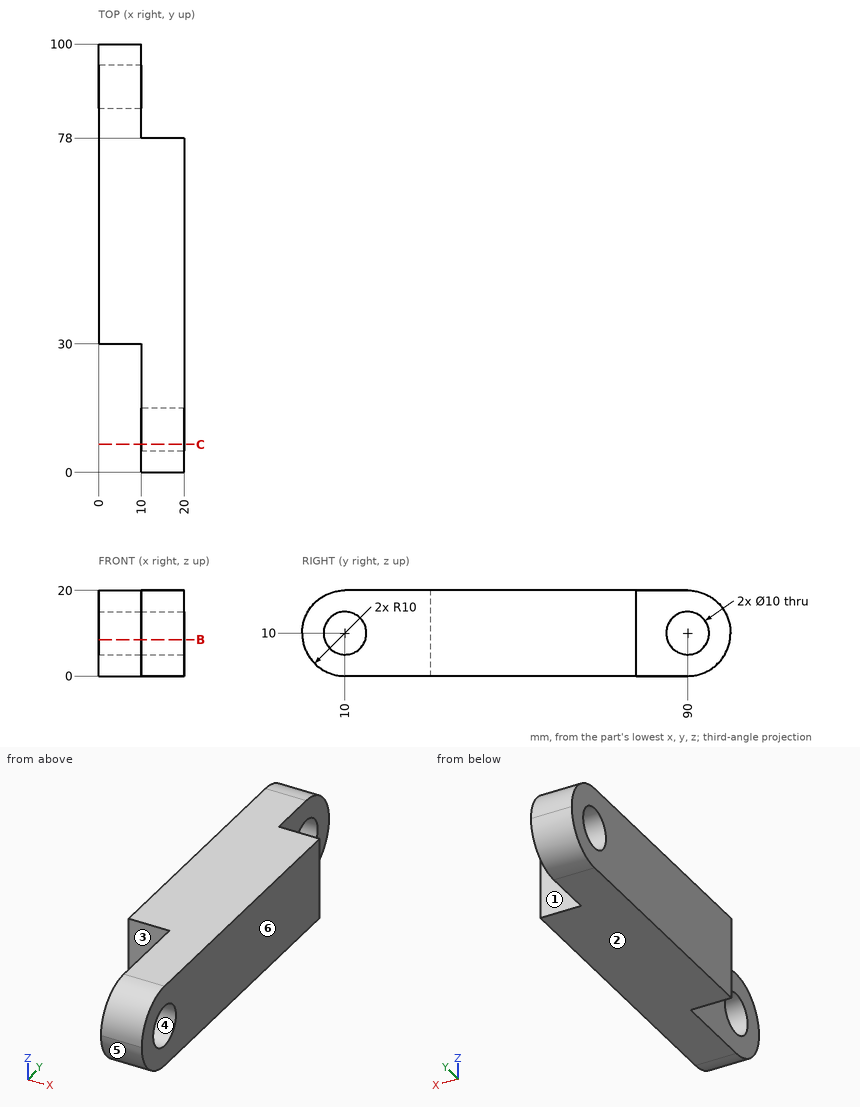
Can you work these out from the drawing? Everything is in mm from the part's minimum corner. A direction names the side the tool comes from. Round coordinates to 2 decimals unless told otherwise and drop trailing zeros. Order: outer loops, then holes, each group sorted by start corner. A loop starts at its lowest first (then second) coordinate and runs counter-clockwise, first axis right, second up. Notation, with made-up numbers: M -31,-37 L -7,-37 A25 cw -7,-21 Z; hole C -30,30.5 d3. An arc over 180 degrees is marked long. Answer as CSV lines item,"result".
Item 1: Imagine slicing it at C-C on y = 6.5. List the corners of the cut face in (x, z) for me.
From the geometry:
outline,"M 10,0.63 L 20,0.63 L 20,6.43 L 10,6.43 Z; M 10,13.57 L 20,13.57 L 20,19.37 L 10,19.37 Z"
Item 2: Please list where these lines run through material, in increasing order: L1, parallel to Z at x = 13.5, y = 10; L2, parallel to X at y = 82.5, z = 11.25; L3, parallel to Y at x = 4.75, z = 13. Write a range as [from, to].
From the geometry:
L1,"[0, 5], [15, 20]"
L2,"[0, 10]"
L3,"[30, 86], [94, 99.54]"
Item 3: For pin 1 (6 mm diameter, centred on y = 94, z = 13.5, fed in from +X); pin 2 (5 mm diameter, centred on x = 4, z = 15, fed in from -Y); pin 3 (8 mm diameter, centred on x = 6.5, z = 3.5, fed in from +Y), each with a flat end and sliding along its axis, tell me the tip position at first contact or that it passes through.
From the geometry:
pin 1,"x = 10"
pin 2,"y = 30"
pin 3,"y = 99.68"
Item 4: We'd pull the mould along Z, two halves only. Please class the marked faces 4, 5 and 6: +Z half, -Z half, draft (parallel to the pull), parting line (faces both ways), or undercut.
From the geometry:
face 4,"undercut"
face 5,"-Z half"
face 6,"draft"
Item 5: Which directions (+Z, -Z, +X, -X, +Y, -Y) give clear straight access to the entire face, cutting with the end or side of a thin tool? Please do the marked faces 1, 2 and 3.
From the geometry:
face 1,"+Z, -Z, +X, +Y"
face 2,"-Z, +X, -X, +Y, -Y"
face 3,"+Z, -Z, -X, -Y"
Item 6: Imagine slicing it at B-B on z = 8.5. List the corners of the cut face in (x, y) for me, and give its area (3 significant figures).
From the geometry:
outline,"M 0,30 L 10,30 L 10,14.77 L 20,14.77 L 20,78 L 10,78 L 10,85.23 L 0,85.23 Z; M 0,94.77 L 10,94.77 L 10,99.89 L 0,99.89 Z; M 10,0.11 L 20,0.11 L 20,5.23 L 10,5.23 Z"
area,"1,290 mm2"
